Design review of the part built by this model. Coordinates are the model's own, in mm. Give positions to 0.01 mm unless a question says otherwise; leave off trailing zeros. Loops run counter-clockwise (first coordinate to the right, second up) from the corner with the lowest first, then second, coordinate; pieces in that order, holes last.
Autodesk Inventor part; units mm, degrees
ref_plane "YZ Plane" through (0, 0, 0) normal (1, 0, 0) x (0, 1, 0)
ref_plane "XZ Plane" through (0, 0, 0) normal (0, 1, 0) x (-1, 0, 0)
ref_plane "XY Plane" through (0, 0, 0) normal (0, 0, 1) x (1, 0, 0)
sketch "スケッチ1" plane through (0, 0, 0) normal (0, 0, 1) x (1, 0, 0)
  line L0 (0, 0) -> (80, 0)
  line L1 (80, 0) -> (80, 60)
  line L2 (80, 60) -> (0, 60)
  line L3 (0, 60) -> (0, 0)
  dimension "d0" = 80
  dimension "d1" = 60
extrude "押し出し1" add sketch "スケッチ1" along normal blind 3
sketch "スケッチ2" plane through (0, 0, 3) normal (0, 0, 1) x (1, 0, 0)
  point P0 (0, 0)
sketch "スケッチ3" plane through (0, 0, 3) normal (0, 0, 1) x (1, 0, 0)
  line L0 (0, 0) -> (80, 0)
  line L1 (15, 0) -> (15, 60) construction
  line L2 (15, 0) -> (75, 0) construction
  line L3 (0, 60) -> (0, 0)
  circle A0 centre (7.5, 30) radius 1.6
  circle A1 centre (7.5, 40) radius 1.6
  circle A2 centre (7.5, 20) radius 1.6
  line L4 (80, 60) -> (0, 60)
  line L5 (40, 60) -> (40, 0) construction
  circle A3 centre (72.5, 30) radius 1.6
  circle A4 centre (72.5, 40) radius 1.6
  circle A5 centre (72.5, 20) radius 1.6
  point P0 (0, 30)
  dimension "d4" = 60
  dimension "d5" = 90
  dimension "d6" = 15
  dimension "d7" = 3.2
  dimension "d8" = 7.5
  dimension "d9" = 30
  dimension "d10" = 3.2
  dimension "d11" = 3.2
  dimension "d12" = 10
  dimension "d13" = 10
  dimension "d14" = 40
hole "穴1" at (7.5, 40, 3) at (7.5, 30, 3) at (7.5, 20, 3) at (72.5, 40, 3) at (72.5, 30, 3) at (72.5, 20, 3) direction (0, 0, -1) diameter 3.2 end through all
sketch "スケッチ4" plane through (0, 0, 3) normal (0, 0, 1) x (1, 0, 0)
  circle A0 centre (40, 30) radius 7.5
  line L0 (80, 60) -> (0, 60)
  line L1 (80, 0) -> (80, 60)
  point P0 (0, 0)
  dimension "d22" = 15
  dimension "d23" = 30
  dimension "d24" = 40
extrude "押し出し2" cut sketch "スケッチ4" against normal blind 3
sketch "スケッチ5" plane through (0, 0, 3) normal (0, 0, 1) x (1, 0, 0)
  point P0 (0, 0)
sketch "スケッチ6" plane through (0, 0, 3) normal (0, 0, 1) x (1, 0, 0)
  circle A0 centre (40, 30) radius 7.5
  circle A1 centre (40, 30) radius 12.1
  point P0 (0, 0)
  dimension "d27" = 24.2
extrude "押し出し3" cut sketch "スケッチ6" against normal blind 3
sketch "スケッチ7" plane through (0, 0, 3) normal (0, 0, 1) x (1, 0, 0)
  circle A0 centre (40, 30) radius 12.1
  line L0 (0, 0) -> (80, 0)
  point P0 (62.851, 30)
  point P1 (17.149, 30)
  dimension "d30" = 22.851
  dimension "d31" = 22.851
  dimension "d32" = 30
  dimension "d33" = 30
hole "穴2" at (17.149, 30, 3) at (62.851, 30, 3) direction (0, 0, -1) diameter 3.2 end through all
fillet "フィレット1" radius 6 4 edges at (0, 60, 1.5) (80, 60, 1.5) (80, 0, 1.5) (0, 0, 1.5)
sketch "スケッチ8" plane through (0, 0, 3) normal (0, 0, 1) x (1, 0, 0)
  point P0 (0, 0)
properties part number "射出_エンコーダー固定" material "アルミニウム 6061"
Q1. Take a section at D-D (z = 0.75). Give the number of separate pieces and of enclosed holes in the cut face, plus the area to 3 significant figures.
Results:
separate pieces: 1
enclosed holes: 9
area: 4,240 mm2
Q2. Draft analysis for pull direction X (two halves, no side actions). For faces 1 (the face through (9.06, 40.35, 1.48)), 2 (the face through (78.196, 1.711, 1.521)), 3 (the face through (39, 44, 3)), state which applies: pulls with the +X half, pulls with the -X half, needs draft (parallel to the pull), parting line crosses it, or undercut.
Results:
face 1: undercut
face 2: pulls with the +X half
face 3: needs draft
Q3. Take a section at B-B (x = 72.5). Give the boundary of the cut face in (y, z), plus the area to 3 significant figures.
Results:
outline: (0, 0) - (18.4, 0) - (18.4, 3) - (0, 3) - close; (21.6, 0) - (28.4, 0) - (28.4, 3) - (21.6, 3) - close; (31.6, 0) - (38.4, 0) - (38.4, 3) - (31.6, 3) - close; (41.6, 0) - (60, 0) - (60, 3) - (41.6, 3) - close
area: 151 mm2
Q4. Take a section at C-C (y = 20). Give the boundary of the cut face in (x, z).
Results:
outline: (0, 0) - (5.9, 0) - (5.9, 3) - (0, 3) - close; (9.1, 0) - (33.19, 0) - (33.19, 3) - (9.1, 3) - close; (46.81, 0) - (70.9, 0) - (70.9, 3) - (46.81, 3) - close; (74.1, 0) - (80, 0) - (80, 3) - (74.1, 3) - close
Q5. Take a section at A-A (y = 30). Give the boundary of the cut face in (x, z).
Results:
outline: (0, 0) - (5.9, 0) - (5.9, 3) - (0, 3) - close; (9.1, 0) - (15.55, 0) - (15.55, 3) - (9.1, 3) - close; (18.75, 0) - (27.9, 0) - (27.9, 3) - (18.75, 3) - close; (52.1, 0) - (61.25, 0) - (61.25, 3) - (52.1, 3) - close; (64.45, 0) - (70.9, 0) - (70.9, 3) - (64.45, 3) - close; (74.1, 0) - (80, 0) - (80, 3) - (74.1, 3) - close
Q6. Wall thickness on line 1 (Y direction, x = 72.5, z = 1.1); line 2 (X direction, y = 19.5, z = 2.4); line 3 (Y direction, x = 73, z = 2.85): over which ranges is each line inside the solid? List them lowest first.
Results:
line 1: y = 0 to 18.4, 21.6 to 28.4, 31.6 to 38.4, 41.6 to 60
line 2: x = 0 to 5.98, 9.02 to 33.99, 46.01 to 70.98, 74.02 to 80
line 3: y = 0 to 18.48, 21.52 to 28.48, 31.52 to 38.48, 41.52 to 60
